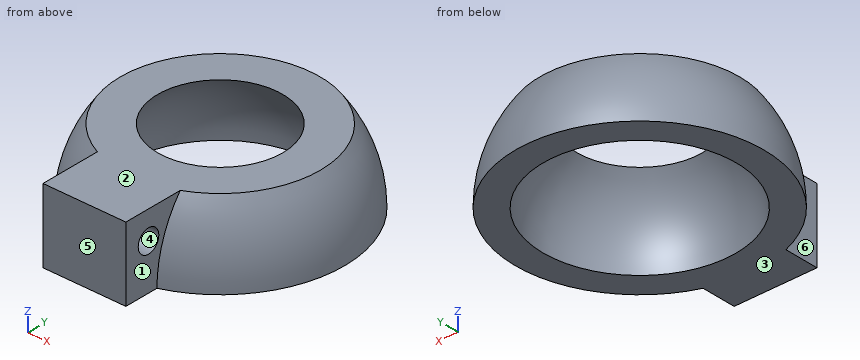
```python
from build123d import *

# Parameters (mm, degrees)
SKETCH4_W                = 9
SKETCH4_H                = 8
BASEBOSS_DEPTH           = 3
BOSS_EXTRUDE3_REACH      = 37.383
BOSS_EXTRUDE3_END_RADIUS = 13.5
SKETCH4_5_W              = 9
SKETCH4_5_H              = 8
CUT_EXTRUDE2_REACH       = 94.415
SKETCH7_R                = 1.25


with BuildPart() as part:
    # Sketch4 → BaseBoss (new body)
    with BuildSketch(Plane(origin=(0, 60.25, 0), x_dir=(1, 0, 0), z_dir=(0, 1, 0))):
        with Locations((-3.25, 4.451253904)):
            Rectangle(SKETCH4_W, SKETCH4_H)
    extrude(amount=BASEBOSS_DEPTH)



with BuildPart() as body_2:
    # Sketch5 → CoverRevolve (revolve)
    with BuildSketch(Plane.ZY.offset(3.25), mode=Mode.PRIVATE) as coverrevolve_sk:
        with BuildLine():
            Line((-8.451253904, 63.25), (-8.451253904, 66.25))
            ThreePointArc((-8.451253904, 66.25), (-4.044311663, 67.219582376), (-0.451253904, 69.949264746))
            Line((-0.451253904, 69.949264746), (-0.451253904, 65.875718415))
            ThreePointArc((-0.451253904, 65.875718415), (-4.24131337, 63.923215496), (-8.451253904, 63.25))
        make_face()
    revolve(coverrevolve_sk.sketch.rotate(Axis((-3.25, 76.75, -0.451253904), (0, 0, -1)), 270), axis=Axis((-3.25, 76.75, -0.451253904), (0, 0, -1)))


with BuildPart() as part_1:
    add(part.part)

    add(body_2.part)  # Boss-Extrude3 merges body 2
    # Boss-Extrude3: up to this sphere (the profile starts outside it)
    boss_extrude3_end = Location((-3.25, 76.75, -8.451253904)) * Sphere(BOSS_EXTRUDE3_END_RADIUS, mode=Mode.PRIVATE)
    # Sketch4<5> → Boss-Extrude3 (add, up to the surface)
    with BuildSketch(Plane(origin=(0, 60.25, 0), x_dir=(1, 0, 0), z_dir=(0, 1, 0)), mode=Mode.PRIVATE) as boss_extrude3_sk1:
        with Locations((-3.25, 4.451253904)):
            Rectangle(SKETCH4_5_W, SKETCH4_5_H)
    boss_extrude3_tool1 = extrude(boss_extrude3_sk1.sketch, amount=BOSS_EXTRUDE3_REACH, mode=Mode.PRIVATE) - boss_extrude3_end
    add(boss_extrude3_tool1.solids().sort_by_distance((-3.25, 60.25, -4.451254))[0])

    # Sketch7 → Cut-Extrude2 (cut, up to next)
    with BuildSketch(Plane(origin=(1.25, 0, 0), x_dir=(0, 0, -1), z_dir=(1, 0, 0)), mode=Mode.PRIVATE) as cut_extrude2_sk1:
        with Locations((3.496708449, 63)):
            Circle(SKETCH7_R)
    cut_extrude2_tool1 = extrude(cut_extrude2_sk1.sketch, amount=-CUT_EXTRUDE2_REACH, mode=Mode.PRIVATE) & part_1.part
    add(cut_extrude2_tool1.solids().sort_by_distance((1.25, 63, -3.496708))[0], mode=Mode.SUBTRACT)


solid = part_1.part
```
Could you check a few things on this model? Use its own coordinates, in mm. Face numbers are marked on the shaded views. A direction names the side the tool comes from. Coordinates: 2 decimals unless noted, no trailing zeros. Write each loop counter-clockwise with the first axis right and the second up, starting at its lowest first coordinate (ties: lowest second). Pieces come first, ordered by that corner, then holes. Notation, with made-up numbers: (60.25, 15.25) -> (117.25, 15.25) arc R25 cw to (117.25, 43.25) -> close; hole circle Ø4 at (-10, 56). An arc over 180 degrees is marked (long way). Write item = value, one per line. Start each with the question number.
(1) I want a section at B-B (y = 63). Please give me the cut outline in (x, z).
(2) I need wall thicknesses on line 1 (Y direction, x = -6.25, z = -3.5); line 2 (Y direction, x = -1.75, z = -4.5); line 3 (Y direction, x = 2, z = -5.25). Which ranges of each line are inside material? Lowest first, please. Write a range as [from, to].
(3) I want a section at A-A (x = -5.5). Please give me the cut outline in (y, z).
(4) We'd pull the mould along Z, two halves only. Please class the marked faces 1, 2, 3 and 4: released by +Z, released by -Z, zero draft, split by the parting line, or undercut.
(5) Will these pins go through, and if not, where does the flat tip stop? pin 1 (3.5 mm diameter, centred on y = 63.5, z = -5.5, fed in from -X); pin 2 (2 mm diameter, centred on y = 63, z = -3.5, fed in from -X); pin 3 (2 mm diameter, centred on y = 84, z = -5.5, fed in from -X); pin 4 (1 mm diameter, centred on y = 68, z = -6, fed in from -X).
(6) I want a section at D-D (x = 2.75). Please give me the cut outline in (y, z), plus the area to 3 significant figures.
(7) I want a section at C-C (z = -3.75). Please give me the cut outline in (x, y).
(8) Which directions (+Z, -Z, +X, -X, +Y, -Y) give clear straight access to the entire face, cutting with the end or side of a thin tool? Please do the marked faces 5 and 6.
Result set:
q1.outline = (-7.75, -8.45) -> (1.25, -8.45) -> (1.25, -4.75) -> (-7.75, -4.75) -> close; (-7.75, -2.25) -> (1.25, -2.25) -> (1.25, -0.45) -> (-7.75, -0.45) -> close
q2.line_1 = [60.25, 61.75], [64.25, 67.99], [85.51, 88.95]
q2.line_2 = [60.25, 62.25], [63.75, 67.14], [86.36, 89.57]
q2.line_3 = [64.73, 68.24], [85.26, 88.77]
q3.outline = (60.25, -8.45) -> (66.49, -8.45) arc R10.26 cw to (70.33, -0.45) -> (60.25, -0.45) -> close; (83.17, -0.45) arc R10.26 cw to (87.01, -8.45) -> (90.06, -8.45) arc R13.31 ccw to (87.39, -0.45) -> close; hole circle Ø2.5 at (63, -3.5)
q4.face_1 = zero draft
q4.face_2 = released by +Z
q4.face_3 = released by -Z
q4.face_4 = undercut
q5.pin_1 = -9.76
q5.pin_2 = through
q5.pin_3 = -14.9
q5.pin_4 = -13.67
q6.outline = (64.66, -8.45) -> (68.13, -8.45) arc R8.62 cw to (73.55, -0.45) -> (67.68, -0.45) arc R12.09 ccw to start; (79.95, -0.45) arc R8.62 cw to (85.37, -8.45) -> (88.84, -8.45) arc R12.09 ccw to (85.82, -0.45) -> close
q6.area = 64.3 mm2
q7.outline = (-7.75, 60.25) -> (1.25, 60.25) -> (1.25, 61.78) -> (-7.75, 61.78) -> close; (-7.75, 64.22) -> (1.25, 64.22) -> (1.25, 64.92) arc R12.65 ccw (long way) to (-7.75, 64.92) -> close; hole circle Ø18.78 at (-3.25, 76.75)
q8.face_5 = +Z, -Z, +X, -X, -Y
q8.face_6 = +Z, -X, -Y
